Drawing for the job (mm, zero at the part's lowest x, y, z). Give positions to 0.01 mm unless a question says otherwise; leave off trailing zeros. Order: outer loops, then holes, each group sorted by start corner. A loop starts at its lowest first (then second) coordinate and runs counter-clockwise, first axis right, second up. Notation, with made-up numbers: (15, -23.75) -> (47, -23.75) arc R14 ccw to (47, -0.75) -> close; hole circle Ø1 at (-1, -23.5). An arc over 180 degrees is marked (long way). One line per item, written item: value. Start each with the question number.
(1) Probe line 1 (X direction, y = 1.25, z = 2.75); line 2 (Y direction, x = 172, z = 12.75). List the from-to ranges inside material, lowest first.
(2) Saw through at A-A on y = 4.5. Give the cut face in (x, z), plus the area to 3 significant figures.
(3) Pin check, flat tips, straight feed: pin 1 (1.9 mm diameter, centred on x = 4.5, y = 2.5, fed in from -Z); pin 2 (3 mm diameter, centred on y = 3, z = 6, fed in from -X); pin 3 (1.9 mm diameter, centred on x = 3, y = 4, fed in from +Z). Stop position of each tip, or through.
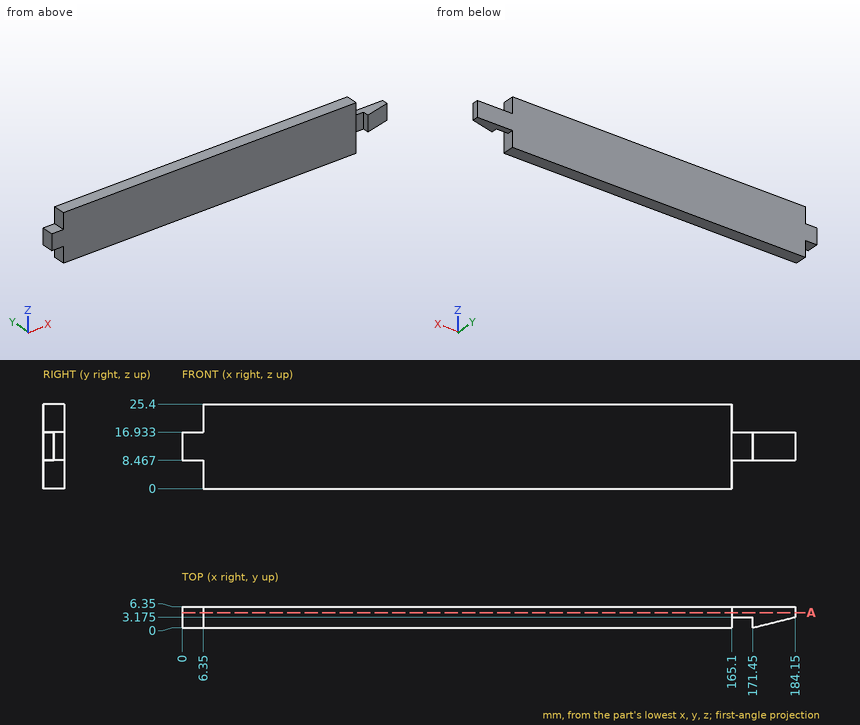
Results below:
1. line 1: x = 6.35 to 165.1
1. line 2: y = 0.14 to 6.35
2. outline: (0, 8.47) -> (6.35, 8.47) -> (6.35, 0) -> (165.1, 0) -> (165.1, 8.47) -> (184.15, 8.47) -> (184.15, 16.93) -> (165.1, 16.93) -> (165.1, 25.4) -> (6.35, 25.4) -> (6.35, 16.93) -> (0, 16.93) -> close
2. area: 4,250 mm²
3. pin 1: stops at z = 8.47
3. pin 2: stops at x = 6.35
3. pin 3: stops at z = 16.93
